CAD build for the part. Positions are in the model's coordinates, mm. A direction names the side the tool comes from. Round coordinates to 2 decimals unless told otherwise and drop trailing zeros. Order: outer loops, then holes, each group sorted by start corner. A loop starts at its lowest first (then second) coordinate and runs counter-clockwise, first axis right, second up. Notation, with made-up numbers: M -28.5,24 L 10.5,24 A13 ccw 10.5,46 Z; hole C 20.5,-17 d1. An arc over 180 degrees is marked long. Answer as CSV lines item,"result". Start each with the question number.
```python
from build123d import *

# Parameters (mm, degrees)
SKETCH1_W           = 12.5
SKETCH1_H           = 13.4
BOSS_EXTRUDE1_DEPTH = 6.5
SKETCH2_R           = 3.5
BOSS_EXTRUDE2_DEPTH = 7
SKETCH3_R           = 3
BOSS_EXTRUDE3_DEPTH = 23
CHAMFER1_SIZE       = 0.5
CUT_EXTRUDE1_DEPTH  = 12
SKETCH5_W           = 0.8
SKETCH5_H           = 10.2
BOSS_EXTRUDE4_DEPTH = 0.5


with BuildPart() as part:
    # Sketch1 → Boss-Extrude1 (new body)
    with BuildSketch(Plane(origin=(0, 0, 0), x_dir=(1, 0, 0), z_dir=(0, 1, 0))):
        Rectangle(SKETCH1_W, SKETCH1_H)
    extrude(amount=-BOSS_EXTRUDE1_DEPTH)

    # Sketch2 → Boss-Extrude2 (add)
    with BuildSketch(Plane(origin=(0, 0, 0), x_dir=(1, 0, 0), z_dir=(0, 1, 0))):
        Circle(SKETCH2_R)
    extrude(amount=BOSS_EXTRUDE2_DEPTH)

    # Sketch3 → Boss-Extrude3 (add)
    with BuildSketch(Plane(origin=(0, 7, 0), x_dir=(1, 0, 0), z_dir=(0, 1, 0))):
        Circle(SKETCH3_R)
    extrude(amount=BOSS_EXTRUDE3_DEPTH)

    # Chamfer1
    chamfer1_edges = [part.edges().sort_by_distance(p)[0] for p in [
        (-3, 30, 0),
    ]]
    chamfer(chamfer1_edges, length=CHAMFER1_SIZE)

    # Sketch4 → Cut-Extrude1 (cut)
    with BuildSketch(Plane(origin=(0, 30, 0), x_dir=(1, 0, 0), z_dir=(0, 1, 0))):
        with BuildLine():
            Line((-2.598076211, -1.5), (2.598076211, -1.5))
            ThreePointArc((2.598076211, -1.5), (0, -3), (-2.598076211, -1.5))
        make_face()
    extrude(amount=-CUT_EXTRUDE1_DEPTH, mode=Mode.SUBTRACT)

    # Sketch5 → Boss-Extrude4 (add)
    with BuildSketch(Plane.XY.offset(6.7)):
        with Locations((-2.5, -5.1)):
            Rectangle(SKETCH5_W, SKETCH5_H)
        with Locations((0, -5.1)):
            Rectangle(SKETCH5_W, SKETCH5_H)
        with Locations((2.5, -5.1)):
            Rectangle(SKETCH5_W, SKETCH5_H)
    extrude(amount=BOSS_EXTRUDE4_DEPTH)


solid = part.part
```
Q1. Tool access for faces 1 (the cylindrical face through (3.233, 3.451, 1.341)), 2 (the flat face through (0, 24, 1.5)), 3 (the flat face through (-1, -3, 6.7)): list every direction of +Z, -Z, +X, -X, +Y, -Y with a clear straight run to the whole face (end or side of a thin tool).
Q2. Drop flat-ended pins along their axis: P1, Ø0.9, axis at x = -2.5, y = -7.5, coming from the -Z side; P2, Ø1.6, axis at x = 1, y = 22.5, coming from the +Z side; P3, Ø5, axis at x = -2.5, y = 14, coming from the +Z side. Give the stop position or say it passes through.
Q3. Probe line 1 along Y through (x, z) = (3.25, 5.25); line 2 along Z through (x, y) = (-0.75, 13); line 3 along Z through (x, y) = (1.5, 20.5). List the from-to ranges inside material, lowest first. Write a range as from..to.
Q4. Band-saw the part on D-D, the plane z = 5.25. Write the cut outline in (x, y), then the cut area to 4 significant figures.
Q5. Mould opens along X. For faces 4 (the flat face through (-3, 0, 3)), 5 (the flat face through (6.25, -3, 0)), 6 (the flat face through (1, -3, 6.7)) say: +X half, -X half, draft (parallel to the pull), parting line (faces both ways), or undercut.
Q6. Band-saw the part on A-A, the plane z = 0. Write the cut outline in (x, y), then the cut area to 3 significant figures.
Q7. Band-saw the part on C-C, the plane x = 0. Write the cut outline in (y, z), then the cut area to 3 significant figures.
Q8. Band-saw the part on B-B, the plane y = -6. Write the cut outline in (x, z), then the cut area to 3 significant figures.
Answer:
1,face 1,"+Y"
1,face 2,"+Z, +X, -X, +Y"
1,face 3,"+Z, +Y, -Y"
2,P1,"stops at z = 6.7"
2,P2,"stops at z = 1.5"
2,P3,"stops at z = 3"
3,line 1,"y = -6.5..0"
3,line 2,"z = -2.9..2.9"
3,line 3,"z = -2.6..1.5"
4,outline,"M -6.25,-6.5 L 6.25,-6.5 L 6.25,0 L -6.25,0 Z"
4,area,"81.25 mm^2"
5,face 4,"draft"
5,face 5,"+X half"
5,face 6,"undercut"
6,outline,"M -6.25,-6.5 L 6.25,-6.5 L 6.25,0 L 3.5,0 L 3.5,7 L 3,7 L 3,29.5 L 2.5,30 L -2.5,30 L -3,29.5 L -3,7 L -3.5,7 L -3.5,0 L -6.25,0 Z"
6,area,"268 mm^2"
7,outline,"M -10.2,6.7 L -6.5,6.7 L -6.5,-6.7 L 0,-6.7 L 0,-3.5 L 7,-3.5 L 7,-3 L 29.5,-3 L 30,-2.5 L 30,1.5 L 18,1.5 L 18,3 L 7,3 L 7,3.5 L 0,3.5 L 0,7.2 L -10.2,7.2 Z"
7,area,"261 mm^2"
8,outline,"M -6.25,-6.7 L 6.25,-6.7 L 6.25,6.7 L 2.9,6.7 L 2.9,7.2 L 2.1,7.2 L 2.1,6.7 L 0.4,6.7 L 0.4,7.2 L -0.4,7.2 L -0.4,6.7 L -2.1,6.7 L -2.1,7.2 L -2.9,7.2 L -2.9,6.7 L -6.25,6.7 Z"
8,area,"169 mm^2"
